Geometry: see drawing. Coordinates: mm, zero at the bounding-box minimum. A direction names the side the tool comes from. Give positions to 0.01 mm unless a question says otherwise; leave off trailing zeros. Loops run counter-clockwise (first coordinate to the right, second up) from the corner with the lowest first, then second, coordinate; pieces in that order, holes last. Notation, with made-up numbers: M 87.5,-31.75 L 139.5,-31.75 A29 cw 139.5,-3.75 Z; hole C 5.25,35.5 d6. An arc over 180 degrees is marked long. Put each result on its own line as item: value.
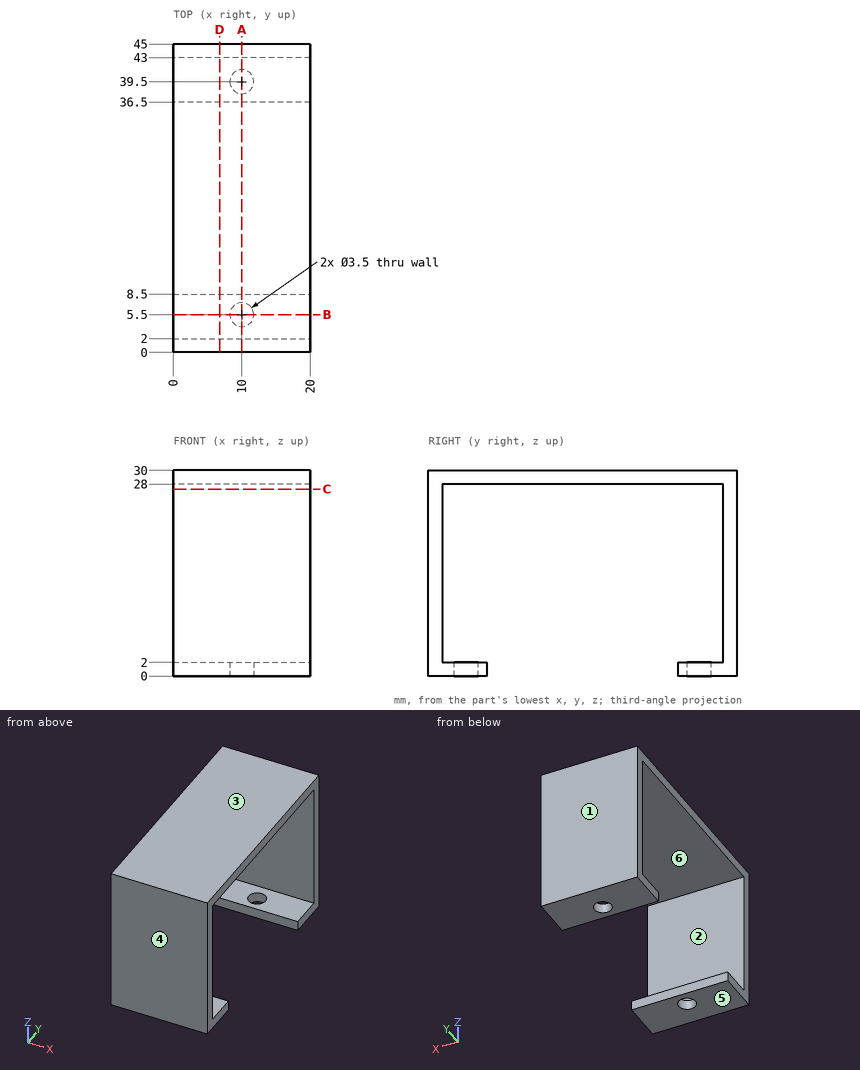
1. Draft query along Y for the marked faces 1, 2, 3 and 4. Return one class per face: pulls with the +Y half, pulls with the -Y half, needs draft (parallel to the pull), parting line crosses it, or undercut.
Found:
face 1: pulls with the +Y half
face 2: undercut
face 3: needs draft
face 4: pulls with the -Y half
2. Section query B-B (y = 5.5). Output: boundary loops of the cut face in (x, z).
Found:
outline: M 0,0 L 8.25,0 L 8.25,2 L 0,2 Z; M 0,28 L 20,28 L 20,30 L 0,30 Z; M 11.75,0 L 20,0 L 20,2 L 11.75,2 Z
3. Section query A-A (x = 10). Output: boundary loops of the cut face in (y, z).
Found:
outline: M 0,0 L 3.75,0 L 3.75,2 L 2,2 L 2,28 L 43,28 L 43,2 L 41.25,2 L 41.25,0 L 45,0 L 45,30 L 0,30 Z; M 7.25,0 L 8.5,0 L 8.5,2 L 7.25,2 Z; M 36.5,0 L 37.75,0 L 37.75,2 L 36.5,2 Z
4. Material intervals for line 1 (Y direction, x = 10, z = 1); line 2 (Z direction, x = 18.75, y = 5); line 3 (X direction, y = 39.5, z = 0.45), sorted ascending. Write a range as from..to.
Found:
line 1: 0..3.75, 7.25..8.5, 36.5..37.75, 41.25..45
line 2: 0..2, 28..30
line 3: 0..8.25, 11.75..20
5. Contact query for a flat-ended pin moving along its axis: P1, Ø10, axis at x = 14.5, y = 24.5, coming from the -Z side. Output: stop coordinate, or through.
Found:
P1: z = 28
6. Section query C-C (z = 27.25). Output: boundary loops of the cut face in (x, y).
Found:
outline: M 0,0 L 20,0 L 20,2 L 0,2 Z; M 0,43 L 20,43 L 20,45 L 0,45 Z
7. Access query for the marked faces 5 and 6. Directions: +Z, -Z, +X, -X, +Y, -Y. A direction counts if a zero-diameter tool reaches every point of the face in a straight line with its end or side. Return the directions, or none.
Found:
face 5: -Z, +X, -X, +Y, -Y
face 6: +X, -X
8. Section query D-D (x = 6.75). Output: boundary loops of the cut face in (y, z), plus the area to 3 significant figures.
Found:
outline: M 0,0 L 8.5,0 L 8.5,2 L 2,2 L 2,28 L 43,28 L 43,2 L 36.5,2 L 36.5,0 L 45,0 L 45,30 L 0,30 Z
area: 228 mm^2
